Can you work these out from the model? Positions are in its coordinate system, mm. A direction names the side the tool comes from. Round coordinates to 2 decimals unless told otherwise and drop trailing zeros. Order: outer loops, then holes, each group sorted by start corner. A loop starts at its lowest first (then second) coordinate and runs counter-clockwise, first axis right, second up. Notation, with made-up numbers: (4.25, 9) - (45.25, 9) arc R14 cw to (45.25, 27) - close; hole circle Ø11 at (-25.5, 38). An arc over 180 degrees is marked (long way). Write item = value, one per line.
from build123d import *

# Parameters (mm, degrees)
SKETCH_1_R      = 1.5
EXTRUDE_1_DEPTH = 4


with BuildPart() as part:
    # 草图1 → 凸台-拉伸1 (new body)
    with BuildSketch(Plane.XY):
        with BuildLine():
            Line((58.445187997, 32.9), (74.5685, 32.9))
            ThreePointArc((74.5685, 32.9), (75.982713562, 32.314213562), (76.5685, 30.9))
            Line((76.5685, 30.9), (76.5685, -30.9))
            ThreePointArc((76.5685, -30.9), (75.982713562, -32.314213562), (74.5685, -32.9))
            Line((74.5685, -32.9), (58.445187997, -32.9))
            ThreePointArc((58.445187997, -32.9), (53.927025417, -33.978889817), (50.383782756, -36.982758621))
            ThreePointArc((50.383782756, -36.982758621), (-62.5, 0), (50.383782756, 36.982758621))
            ThreePointArc((50.383782756, 36.982758621), (53.927025417, 33.978889817), (58.445187997, 32.9))
        make_face()
        with Locations((0, -59)):
            Circle(SKETCH_1_R, mode=Mode.SUBTRACT)
        with Locations((-31.89780823, -49.633958437)):
            Circle(SKETCH_1_R, mode=Mode.SUBTRACT)
        with Locations((-53.668287726, -24.509485767)):
            Circle(SKETCH_1_R, mode=Mode.SUBTRACT)
        with Locations((-58.399465071, 8.396575458)):
            Circle(SKETCH_1_R, mode=Mode.SUBTRACT)
        with Locations((-44.589224887, 38.636783303)):
            Circle(SKETCH_1_R, mode=Mode.SUBTRACT)
        with Locations((-16.622220854, 56.610085443)):
            Circle(SKETCH_1_R, mode=Mode.SUBTRACT)
        with Locations((16.622220854, 56.610085443)):
            Circle(SKETCH_1_R, mode=Mode.SUBTRACT)
        with Locations((44.589224887, 38.636783303)):
            Circle(SKETCH_1_R, mode=Mode.SUBTRACT)
        with Locations((31.89780823, -49.633958437)):
            Circle(SKETCH_1_R, mode=Mode.SUBTRACT)
        with BuildLine():
            Line((58.445187997, -30.9), (74.5685, -30.9))
            Line((74.5685, -30.9), (74.5685, 30.9))
            Line((74.5685, 30.9), (58.445187997, 30.9))
            ThreePointArc((58.445187997, 30.9), (53.0233929, 32.19466778), (48.771501708, 35.799310345))
            ThreePointArc((48.771501708, 35.799310345), (48.095161057, 36.702935617), (47.402080553, 37.593786179))
            ThreePointArc((47.402080553, 37.593786179), (42.321976164, 36.672201101), (43.957155069, 41.569442121))
            ThreePointArc((43.957155069, 41.569442121), (32.708769456, 50.895838736), (19.552432438, 57.253405015))
            ThreePointArc((19.552432438, 57.253405015), (15.777023183, 53.731606522), (14.504974825, 58.735472292))
            ThreePointArc((14.504974825, 58.735472292), (0, 60.499999866), (-14.504974825, 58.735472292))
            ThreePointArc((-14.504974825, 58.735472292), (-15.777023183, 53.731606522), (-19.552432438, 57.253405015))
            ThreePointArc((-19.552432438, 57.253405015), (-32.708769456, 50.895838736), (-43.957155069, 41.569442121))
            ThreePointArc((-43.957155069, 41.569442121), (-42.321976164, 36.672201101), (-47.402080553, 37.593786179))
            ThreePointArc((-47.402080553, 37.593786179), (-55.032735719, 25.132608287), (-59.453249164, 11.205407793))
            ThreePointArc((-59.453249164, 11.205407793), (-55.430000745, 7.969630943), (-60.20190302, 5.998405856))
            ThreePointArc((-60.20190302, 5.998405856), (-59.884197234, -8.610047716), (-56.073356727, -22.716264336))
            ThreePointArc((-56.073356727, -22.716264336), (-50.93939174, -23.263240728), (-53.888046644, -27.501425943))
            ThreePointArc((-53.888046644, -27.501425943), (-45.722849122, -39.619074294), (-34.890569724, -49.425683044))
            ThreePointArc((-34.890569724, -49.425683044), (-30.275885778, -47.110197839), (-30.465116213, -52.269749321))
            ThreePointArc((-30.465116213, -52.269749321), (-17.04481965, -58.049324772), (-2.630273359, -60.44279661))
            ThreePointArc((-2.630273359, -60.44279661), (0, -56), (2.630273359, -60.44279661))
            ThreePointArc((2.630273359, -60.44279661), (17.044819652, -58.049324777), (30.465116213, -52.269749321))
            ThreePointArc((30.465116213, -52.269749321), (30.275885778, -47.110197839), (34.890569724, -49.425683044))
            ThreePointArc((34.890569724, -49.425683044), (42.382249319, -43.174007721), (48.771501708, -35.799310345))
            ThreePointArc((48.771501708, -35.799310345), (53.0233929, -32.19466778), (58.445187997, -30.9))
        make_face(mode=Mode.SUBTRACT)
    extrude(amount=EXTRUDE_1_DEPTH)


solid = part.part
(1) If I drill on line 1 (Y direction, x = 0, z = 2.8); line 2 (Y direction, x = -31, z = 3.7); line 3 (X direction, y = -2, z = 0.9), over which ranges is the centre line in solid material (lowest first)? Write a range as from..to.
Computed:
line_1 = -62.5..-60.5, -57.5..-56, 60.5..62.5
line_2 = -54.27..-50.84, -48.43..-46.77, 51.95..54.27
line_3 = -62.47..-60.47, 74.57..76.57
(2) If we section it at D-D (z = 0.8): State how many separate pieces and enclosed holes the cut face has, plus the area to 3 significant figures.
Computed:
separate_pieces = 1
enclosed_holes = 10
area = 993 mm^2
(3) Will these pins go through, and if not, where does the flat tip stop? P1, Ø4, axis at x = -58.4, y = 8.4, coming from the -Z side; P2, Ø8, axis at x = 47.5, y = 48, coming from the -Z side; P3, Ø1.2, axis at x = 70.5, z = 2, coming from the +Y side; P4, Ø1, axis at y = -12.5, z = 0.5, coming from the -X side.
Computed:
P1 = 0
P2 = through
P3 = 32.9
P4 = -61.34
(4) If we section it at C-C (y = 43.5): Write out the boundary of the cut face in (x, z), plus the area to 3 significant figures.
Computed:
outline = (-44.88, 0) - (-42.05, 0) - (-42.05, 4) - (-44.88, 4) - close; (42.05, 0) - (44.88, 0) - (44.88, 4) - (42.05, 4) - close
area = 22.6 mm^2
(5) On a 3-axis mill with a long thin cutter (end or side, diameter ignored), from which of +Z, -Z, +X, -X, +Y, -Y can I reach the whole of each face in a straight line? I mean faces 5 (the face through (67, 30.9, 2)), 6 (the face through (76.568, 0, 2)). Say none if no direction works.
Computed:
face_5 = +Z, -Z
face_6 = +Z, -Z, +X, +Y, -Y
(6) If we section it at A-A (x = 0): Write out the boundary of the cut face in (y, z).
Computed:
outline = (-62.5, 0) - (-60.5, 0) - (-60.5, 4) - (-62.5, 4) - close; (-57.5, 0) - (-56, 0) - (-56, 4) - (-57.5, 4) - close; (60.5, 0) - (62.5, 0) - (62.5, 4) - (60.5, 4) - close
(7) If we section it at B-B (y = 0): Write out the boundary of the cut face in (x, z), plus the area to 3 significant figures.
Computed:
outline = (-62.5, 0) - (-60.5, 0) - (-60.5, 4) - (-62.5, 4) - close; (74.57, 0) - (76.57, 0) - (76.57, 4) - (74.57, 4) - close
area = 16.0 mm^2
(8) Thinking about a two-plate mould opening in Y: for faces 1 (the face through (-42.3, 36.7, 2)), 2 (the face through (16.427, 58.097, 1.972)), 3 (the face through (-62.46, -2.19, 1.97)), 4 (the face through (53.986, -33.949, 1.972)), which applies, +Y half, -Y half, draft (parallel to the pull), parting line (faces both ways), or undercut?
Computed:
face_1 = undercut
face_2 = undercut
face_3 = parting line
face_4 = -Y half
